Input: part model. Units: mm. Frame: model coordinates. Round coordinates to 2 decimals unless told otherwise and drop trailing zeros. Loops run counter-clockwise (first coordinate to the right, second up) from the corner with the lowest first, then second, coordinate; pieces in that order, holes last.
(1) Cut plane D-D, the plane x = 40.5. Output: boundary loops of the cut face in (y, z), and give its area (3 significant figures).
(2) Cut plane A-A, the plane x = -68.5. Output: boundary loops of the cut face in (y, z), and give its area (3 significant figures).
(3) Line query: line 1 (X direction, y = -6, z = 8); line 2 (X direction, y = -14.5, z = 9); line 3 (Z direction, x = 48.5, y = -23). Output: solid intervals per line, ascending.
(4) First-contact query: pin 1 Ø2.5 at (y, z) = (-16, 20.5) entering from +X; pin 2 Ø5 at (x, y) = (94, -6.5) entering from +Z; pin 3 Ø2.5 at (y, z) = (-12, 20.5) entering from -X; pin 4 Ø10 at (x, z) = (-166.5, 34.5) entering from +Y. Flat tips, straight axial feed; report the tip coordinate or a pass-through.
(5) Cut plane B-B, the plane z = 31. Output: boundary loops of the cut face in (x, y).
(6) Cut plane C-C, the plane y = -4.75. Output: boundary loops of the cut face in (x, z) (1 decimal), and give its area (3 significant figures).
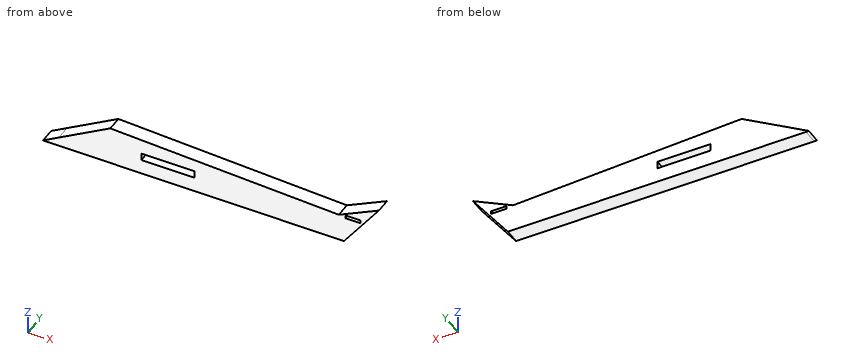
from build123d import *

# Parameters (mm, degrees)
F1_DEPTH  = 25.4
F2_DEPTH  = 25.4
F3_DEPTH  = 25.4
F5_DEPTH  = 25.4
F7_DEPTH  = 25.4
F9_DEPTH  = 25.4
F10_DEPTH = 25.4
F12_DEPTH = 25.4
F15_DEPTH = 25.4
F16_DEPTH = 25.4
F18_DEPTH = 25.4
F20_DEPTH = 25.4
F21_W     = 25.4
F21_H     = 5.08
F22_DEPTH = 25.4


with BuildPart() as f1:
    # F0 (on Front) → F1 (new body)
    with BuildSketch(Plane.XZ):
        with BuildLine():
            ThreePointArc((-248.9374864935, 45.4784197962), (-285.9761731261, 10.2133885569), (-248.9374864935, -25.0516426824))
            Line((-248.9374864935, -25.0516426824), (251.0625135065, -25.0516426824))
            Line((251.0625135065, -25.0516426824), (309.5429599858, 54.4976872176))
            Line((309.5429599858, 54.4976872176), (242.2861912184, 21.3638611095))
            Line((242.2861912184, 21.3638611095), (-248.9374864935, 45.4784197962))
        make_face()
    extrude(amount=F1_DEPTH)

    # F0 (on Front) → F2 (join)
    with BuildSketch(Plane.XZ):
        with BuildLine():
            ThreePointArc((-248.9374864935, 45.4784197962), (-285.9761731261, 10.2133885569), (-248.9374864935, -25.0516426824))
            Line((-248.9374864935, -25.0516426824), (251.0625135065, -25.0516426824))
            Line((251.0625135065, -25.0516426824), (309.5429599858, 54.4976872176))
            Line((309.5429599858, 54.4976872176), (242.2861912184, 21.3638611095))
            Line((242.2861912184, 21.3638611095), (-248.9374864935, 45.4784197962))
        make_face()
    extrude(amount=F2_DEPTH)

    # F0 (on Front) → F3 (join)
    with BuildSketch(Plane.XZ):
        with BuildLine():
            ThreePointArc((-248.9374864935, 45.4784197962), (-285.9761731261, 10.2133885569), (-248.9374864935, -25.0516426824))
            Line((-248.9374864935, -25.0516426824), (251.0625135065, -25.0516426824))
            Line((251.0625135065, -25.0516426824), (309.5429599858, 54.4976872176))
            Line((309.5429599858, 54.4976872176), (242.2861912184, 21.3638611095))
            Line((242.2861912184, 21.3638611095), (-248.9374864935, 45.4784197962))
        make_face()
    extrude(amount=F3_DEPTH)

    # F4 (on face) → F5 (cut)
    with BuildSketch(Plane.XZ.offset(25.4)):
        with BuildLine():
            ThreePointArc((-88.7798070908, 12.3247159645), (-95.8567415785, 6.1623579822), (-88.7798070908, 0))
            Line((-88.7798070908, 0), (0, 0))
            Line((0, 0), (-88.7798070908, 12.3247159645))
        make_face()
    extrude(amount=-F5_DEPTH, mode=Mode.SUBTRACT)

    # F6 (on face) → F7 (cut)
    with BuildSketch(Plane.XZ.offset(25.4)):
        Polygon((0, 0), (-88.7798070908, 12.3247159645), (-88.7798070908, 0), align=None)
        Polygon((0, 12.3247159645), (-88.7798070908, 12.3247159645), (0, 0), align=None)
    extrude(amount=-F7_DEPTH, mode=Mode.SUBTRACT)

    # F11 (on face) → F12 (join)
    with BuildSketch(Plane.XZ.offset(25.4)):
        with BuildLine():
            ThreePointArc((-88.7798070908, 12.3247159645), (-95.8567415785, 6.1623579822), (-88.7798070908, 0))
            Line((-88.7798070908, 0), (-88.7798070908, 12.3247159645))
        make_face()
        with BuildLine():
            Line((-110.1938635111, -10.0966589525), (-88.7798070908, -10.0966589525))
            Line((-88.7798070908, -10.0966589525), (-88.7798070908, 0))
            ThreePointArc((-88.7798070908, 0), (-95.8567415785, 6.1623579822), (-88.7798070908, 12.3247159645))
            Line((-88.7798070908, 12.3247159645), (-88.7798070908, 19.2268192768))
            Line((-88.7798070908, 19.2268192768), (-110.1938635111, 19.2268192768))
            Line((-110.1938635111, 19.2268192768), (-110.1938635111, -10.0966589525))
        make_face()
    extrude(amount=-F12_DEPTH)

    # F13 (on face) → F15 (join)
    with BuildSketch(Plane.XZ.offset(25.4)):
        with BuildLine():
            ThreePointArc((-248.9374864935, 45.4784197962), (-285.9761731261, 10.2133885569), (-248.9374864935, -25.0516426824))
            Line((-248.9374864935, -25.0516426824), (-130.9048912587, 39.6841063828))
            Line((-130.9048912587, 39.6841063828), (-248.9374864935, 45.4784197962))
        make_face()
    extrude(amount=F15_DEPTH)

    # F16 (cut): a face of the model
    f16_faces = [f1.faces().sort_by_distance(p)[0] for p in [
        (-227.9648580508, -50.8, 16.7633050422),
    ]]
    extrude(f16_faces, amount=-F16_DEPTH, mode=Mode.SUBTRACT)

    # F17 (on face) → F18 (cut)
    with BuildSketch(Plane.XZ.offset(25.4)):
        Polygon((-310.474216938, -22.743826732), (-255.3424239159, -25.8090943098), (-138.7038677931, 41.4615124464), (-278.6701321602, 55.0241321325), align=None)
    extrude(amount=-F18_DEPTH, mode=Mode.SUBTRACT)

    # F19 (on face) → F20 (cut)
    with BuildSketch(Plane.XZ.offset(25.4)):
        Polygon((-265.600413084, -31.8100675941), (-141.2684768438, 40.1715748012), (-274.7080028057, 68.8641965389), (-321.2986290455, 3.4738616087), align=None)
    extrude(amount=-F20_DEPTH, mode=Mode.SUBTRACT)

    # F21 (on face) → F22 (cut)
    with BuildSketch(Plane.XZ.offset(25.4)):
        with Locations((266.2754654884, 21.6490322659)):
            Rectangle(F21_W, F21_H)
    extrude(amount=-F22_DEPTH, mode=Mode.SUBTRACT)


with BuildPart() as f9:
    # F8 (on face) → F9 (new body)
    with BuildSketch(Plane.XZ.offset(25.4)):
        with BuildLine():
            Line((-88.7798070908, 0), (-88.7798070908, 12.3247159645))
            ThreePointArc((-88.7798070908, 12.3247159645), (-95.8567415785, 6.1623579822), (-88.7798070908, 0))
        make_face()
    extrude(amount=F9_DEPTH)

    # F10 (cut): a face of the model
    f10_faces = [f9.faces().sort_by_distance(p)[0] for p in [
        (-91.8199479987, -50.8, 6.1623579822),
    ]]
    extrude(f10_faces, amount=-F10_DEPTH, mode=Mode.SUBTRACT)


solid = f1.part
Reported:
1. outline: (-25.4, -25.05) - (0, -25.05) - (0, 31.27) - (-25.4, 31.27) - close
1. area: 1,430 mm2
2. outline: (-25.4, -25.05) - (0, -25.05) - (0, 0) - (-25.4, 0) - close; (-25.4, 12.32) - (0, 12.32) - (0, 36.62) - (-25.4, 36.62) - close
2. area: 1,250 mm2
3. line 1: x = -196.72 to -88.78, 0 to 275.36
3. line 2: x = -194.99 to -88.78, 0 to 276.1
3. line 3: z = -25.05 to 30.88
4. pin 1: stops at x = 285.47
4. pin 2: stops at z = 28.77
4. pin 3: stops at x = -177.22
4. pin 4: passes through
5. outline: (-156.84, -25.4) - (45.99, -25.4) - (45.99, 0) - (-156.84, 0) - close; (261.85, -25.4) - (292.27, -25.4) - (292.27, 0) - (261.85, 0) - close
6. outline: (-253.8, -25) arc R35.3 ccw to (-248.9, -25.1) - (251.1, -25.1) - (309.5, 54.5) - (242.3, 21.4) - (-140.9, 40.2) - (-227.1, -9.5) - close; hole (-88.8, 0) - (0, 0) - (0, 12.3) - (-88.8, 12.3) - close; hole (253.6, 19.1) - (279, 19.1) - (279, 24.2) - (253.6, 24.2) - close
6. area: 25,800 mm2
